Design review of the part shown in the three views and the two pictorial views. Dimensions are in mm from the part's minimum x, y and z. Round coordinates to 2 decimals unless told otherwise and drop trailing zeros. Loops run counter-clockwise (first coordinate to the right, second up) from the corner with the lowest first, then second, coordinate; pieces in that order, holes last. Notation, with made-up numbers: (-3, 76) -> (33, 76) arc R23 ccw to (33, 107) -> close; hole circle Ø5 at (-14.75, 88.25). An arc over 180 degrees is marked (long way). Use a Markdown table: item, result. Add a question column.
1) Consider section D-D on z = 0.3. Give the boundary of the cut face in (x, y).
2) Wall thickness on probe 1 along X at (y, z) = (5.25, 0.55); probe 2 along Y at (x, z) = (17.5, 0.6); probe 3 along X at (y, z) = (4, 0.2): over which ranges is each line inside the solid? List them lowest first.
3) Consider section B-B on x = 4. Give the boundary of the cut face in (y, z), plus the area to 3 significant figures.
4) Consider section C-C on y = 12. Give the boundary of the cut face in (x, z), plus the area to 3 significant figures.
5) Consider section A-A on y = 5.25. Give the boundary of the cut face in (x, z), plus the area to 3 significant figures.
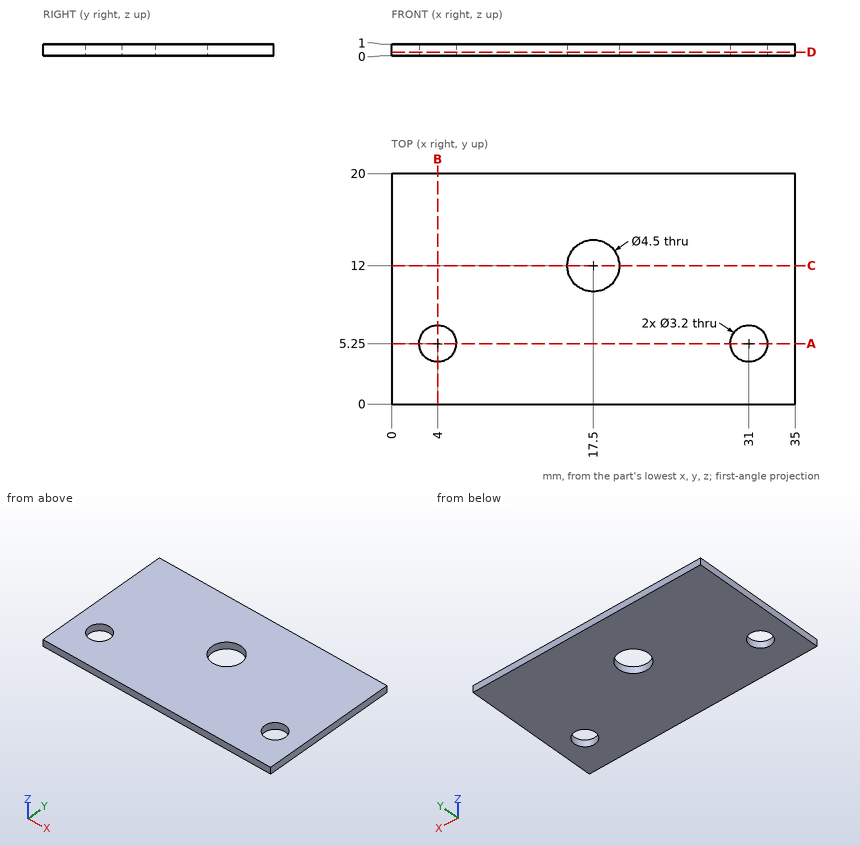
Result set:
| question | item | result |
|---|---|---|
| 1 | outline | (0, 0) -> (35, 0) -> (35, 20) -> (0, 20) -> close; hole circle Ø3.2 at (4, 5.25); hole circle Ø4.5 at (17.5, 12); hole circle Ø3.2 at (31, 5.25) |
| 2 | probe 1 | 0 to 2.4, 5.6 to 29.4, 32.6 to 35 |
| 2 | probe 2 | 0 to 9.75, 14.25 to 20 |
| 2 | probe 3 | 0 to 3, 5 to 30, 32 to 35 |
| 3 | outline | (0, 0) -> (3.65, 0) -> (3.65, 1) -> (0, 1) -> close; (6.85, 0) -> (20, 0) -> (20, 1) -> (6.85, 1) -> close |
| 3 | area | 16.8 mm2 |
| 4 | outline | (0, 0) -> (15.25, 0) -> (15.25, 1) -> (0, 1) -> close; (19.75, 0) -> (35, 0) -> (35, 1) -> (19.75, 1) -> close |
| 4 | area | 30.5 mm2 |
| 5 | outline | (0, 0) -> (2.4, 0) -> (2.4, 1) -> (0, 1) -> close; (5.6, 0) -> (29.4, 0) -> (29.4, 1) -> (5.6, 1) -> close; (32.6, 0) -> (35, 0) -> (35, 1) -> (32.6, 1) -> close |
| 5 | area | 28.6 mm2 |
